Here's the drawing with two shaded views (mm, measured from the low corner). I have some questions. A direction names the side the tool comes from. Coordinates: 2 decimals unless noted, no trailing zeros. Loops run counter-clockwise (first coordinate to the right, second up) from the corner with the lowest first, then second, coordinate; pieces in that order, holes last. Notation, with made-up numbers: (54, 49) -> (100, 49) arc R30 cw to (100, 77) -> close; hole circle Ø8 at (40, 52.25). An arc over 180 degrees is marked (long way). Answer as a JSON object with one key per item and string values. Group by question number.
Q1. I want a section at B-B on y = 19. Write out the boundary of the cut face in (x, z), then the cut area to 3 significant figures.
Q2. I want a section at C-C on x = 30. Write out the boundary of the cut face in (y, z).
Q3. On a 3-axis mill with a long thin cutter (end or side, diameter ignored), from which of +Z, -Z, +X, -X, +Y, -Y can I reach the whole of each face in a straight line? I mean the marked faces 1 and 2. Say none if no direction works.
Q4. I need wall thicknesses on line 1 (Y direction, x = 34, z = 11.75); line 2 (Z direction, x = 36.5, y = 9); line 3 (Y direction, x = 35, z = 8.5). Which ranges of each line are inside material? Lowest first, please.
Q5. I want a section at A-A on z = 4. Write out the boundary of the cut face in (x, y), then the cut area to 3 significant figures.
Q6. I want a section at D-D on z = 27. Write out the boundary of the cut face in (x, y).
Q7. I'm going to push flat-ended pins straight in: pin 1 (5 mm diameter, centred on x = 4, y = 4, fed in from +Z); pin 2 (3 mm diameter, centred on x = 16, z = 26, fed in from -Y). Where does each tip first touch, or does it pass through?
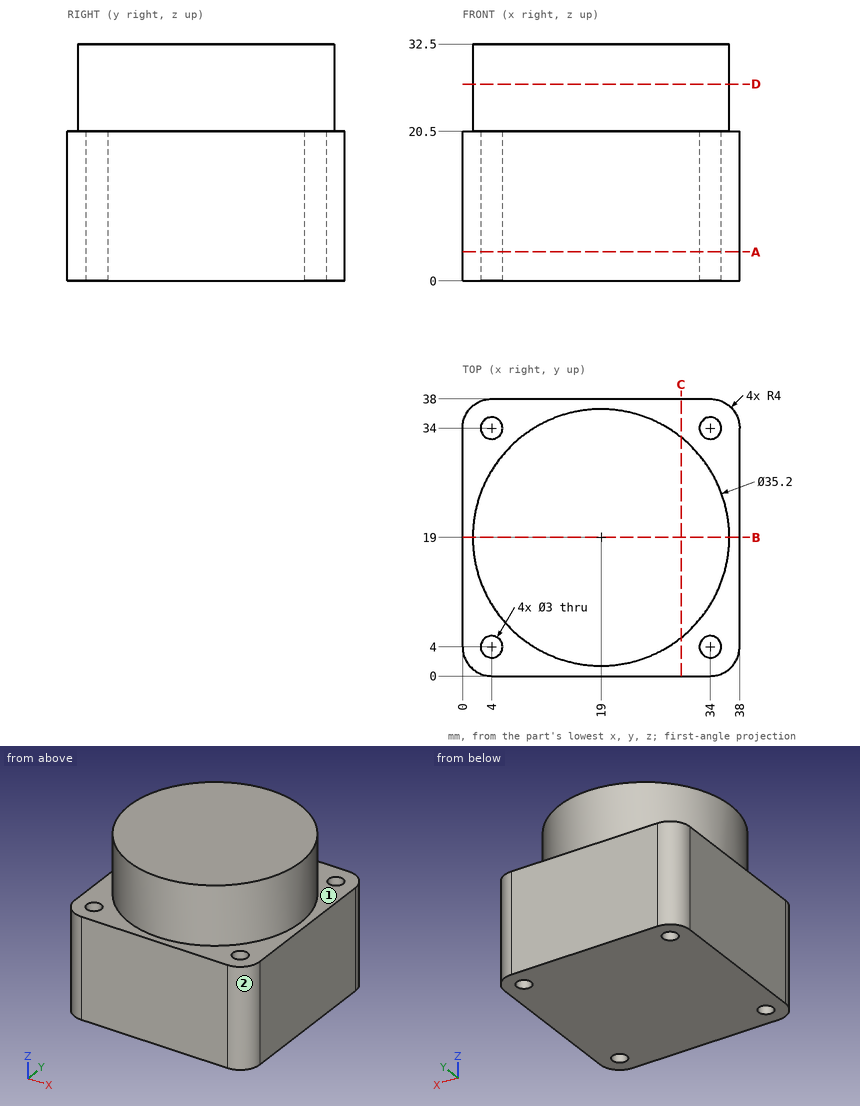
Result set:
{
 "1": {"outline": "(0, 0) -> (38, 0) -> (38, 20.5) -> (36.6, 20.5) -> (36.6, 32.5) -> (1.4, 32.5) -> (1.4, 20.5) -> (0, 20.5) -> close", "area": "1,200 mm²"},
 "2": {"outline": "(0, 0) -> (38, 0) -> (38, 20.5) -> (32.74, 20.5) -> (32.74, 32.5) -> (5.26, 32.5) -> (5.26, 20.5) -> (0, 20.5) -> close"},
 "3": {"face 1": "+Z", "face 2": "+Z, -Z, +X, -Y"},
 "4": {"line 1": "y = 0 to 2.5, 5.5 to 32.5, 35.5 to 38", "line 2": "z = 0 to 20.5", "line 3": "y = 0.13 to 2.88, 5.12 to 32.88, 35.12 to 37.87"},
 "5": {"outline": "(0, 4) arc R4 ccw to (4, 0) -> (34, 0) arc R4 ccw to (38, 4) -> (38, 34) arc R4 ccw to (34, 38) -> (4, 38) arc R4 ccw to (0, 34) -> close; hole circle Ø3 at (4, 4); hole circle Ø3 at (4, 34); hole circle Ø3 at (34, 4); hole circle Ø3 at (34, 34)", "area": "1,400 mm²"},
 "6": {"outline": "circle Ø35.2 at (19, 19)"},
 "7": {"pin 1": "stops at z = 20.5", "pin 2": "stops at y = 1.46"}
}
